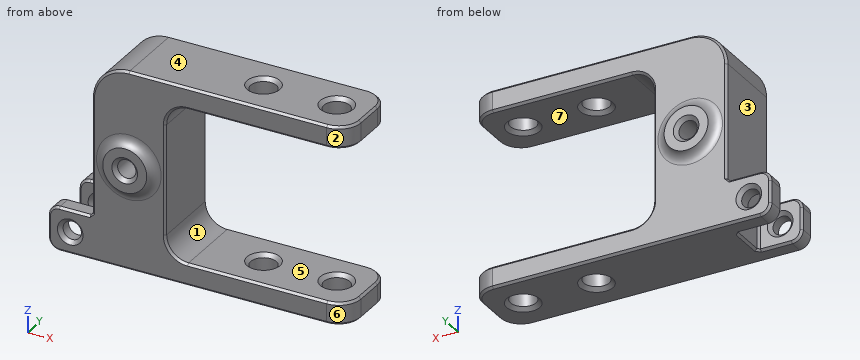
```python
from build123d import *

# Parameters (mm, degrees)
EXTRUDE_1_DEPTH     = 10
SKETCH_2_R          = 1.75
CUT_EXTRUDE_1_DEPTH = 28
SKETCH_3_W          = 6
SKETCH_3_H          = 5.152186346
CUT_EXTRUDE_2_DEPTH = 8
SKETCH_4_R          = 1.25
CUT_EXTRUDE_3_DEPTH = 11
FILLET_1_R          = 3
FILLET_2_R          = 5
FILLET_3_R          = 1.5
SKETCH_5_R          = 3
EXTRUDE_2_DEPTH     = 1
EXTRUDE_START       = 1
SKETCH_6_R          = 3
EXTRUDE_3_DEPTH     = 1
FILLET_4_R          = 1.5
SKETCH_7_R          = 1.25
CUT_EXTRUDE_4_DEPTH = 17
CHAMFER_1_SIZE      = 0.5
FILLET_5_R          = 3
CHAMFER_2_SIZE      = 0.3


with BuildPart() as part:
    # 草图1 → 凸台-拉伸1 (new body)
    with BuildSketch(Plane(origin=(0, 0, 0), x_dir=(1, 0, 0), z_dir=(0, 1, 0))):
        Polygon((23.273216446, 11.883138654), (23.273216446, 8.883138654), (-1.726783554, 8.883138654), (-1.726783554, -12.116861346), (23.273216446, -12.116861346), (23.273216446, -15.116861346), (-11.726783554, -15.116861346), (-11.726783554, 5.883138654), (-17.726783554, 5.883138654), (-17.726783554, 11.883138654), (-11.726783554, 11.883138654), align=None)
    extrude(amount=EXTRUDE_1_DEPTH)

    # 草图2 → 切除-拉伸1 (cut)
    with BuildSketch(Plane(origin=(0, 0, -11.883138654), x_dir=(-1, 0, 0), z_dir=(0, 0, -1))):
        with Locations((-18.858625261, 5)):
            Circle(SKETCH_2_R)
        with Locations((-8.858625261, 5)):
            Circle(SKETCH_2_R)
    extrude(amount=-CUT_EXTRUDE_1_DEPTH, mode=Mode.SUBTRACT)

    # 草图3 → 切除-拉伸2 (cut)
    with BuildSketch(Plane.XY.offset(-5.883138654)):
        with Locations((-14.726783554, 4.923906827)):
            Rectangle(SKETCH_3_W, SKETCH_3_H)
    extrude(amount=-CUT_EXTRUDE_2_DEPTH, mode=Mode.SUBTRACT)

    # 草图4 → 切除-拉伸3 (cut)
    with BuildSketch(Plane(origin=(0, 10, 0), x_dir=(1, 0, 0), z_dir=(0, 1, 0))):
        with Locations(Location((-14.726783554, 8.883138654, 0), (0, 0, 270))):
            Circle(SKETCH_4_R)
    extrude(amount=-CUT_EXTRUDE_3_DEPTH, mode=Mode.SUBTRACT)

    # 圆角1
    fillet_1_edges = [part.edges().sort_by_distance(p)[0] for p in [
        (23.273216446, 0, -10.383138654),
        (23.273216446, 0, 13.616861346),
        (23.273216446, 10, 13.616861346),
        (23.273216446, 10, -10.383138654),
    ]]
    fillet(fillet_1_edges, radius=FILLET_1_R)

    # 圆角2
    fillet_2_edges = [part.edges().sort_by_distance(p)[0] for p in [
        (-11.726783554, 5, 15.116861346),
    ]]
    fillet(fillet_2_edges, radius=FILLET_2_R)

    # 圆角3
    fillet_3_edges = [part.edges().sort_by_distance(p)[0] for p in [
        (-17.726783554, 8.75, -5.883138654),
        (-17.726783554, 8.75, -11.883138654),
        (-17.726783554, 1.173906827, -11.883138654),
        (-17.726783554, 1.173906827, -5.883138654),
    ]]
    fillet(fillet_3_edges, radius=FILLET_3_R)

    # 草图5 → 凸台-拉伸2 (add)
    with BuildSketch(Plane.XZ):
        with Locations(Location((-6.726783554, 2.116861346, 0), (0, 0, 90))):
            Circle(SKETCH_5_R)
    extrude(amount=EXTRUDE_2_DEPTH)

    # 草图6 → 凸台-拉伸3 (add)
    with BuildSketch(Plane(origin=(0, 10, 0), x_dir=(1, 0, 0), z_dir=(0, 1, 0)).offset(EXTRUDE_START)):
        with Locations(Location((-6.726783554, -2.116861346, 0), (0, 0, 270))):
            Circle(SKETCH_6_R)
    extrude(amount=-EXTRUDE_3_DEPTH)

    # 圆角4
    # the kernel refuses this fillet: 1.5 mm, written as the material it adds along each edge
    with BuildSketch(Plane(origin=(-6.726783554, 0, 2.116861346), x_dir=(0, 0, 1), z_dir=(1, 0, 0))) as fillet_4_piece_1:
        with BuildLine():
            CenterArc((4.414213562, 1.5), FILLET_4_R, 199.471220634, 70.528779366)
            Line((3, 1), (2.971715729, 0.99))
            ThreePointArc((2.971715729, 0.99), (2.97, 0.5), (2.97, 0))
            Line((2.97, 0), (3, -0.03))
            Line((3, -0.03), (4.414213562, -0.03))
            Line((4.414213562, -0.03), (4.414213562, 0))
        make_face()
    revolve(axis=Axis((-6.726783554, 0, 2.116861346), (0, -1, 0)))
    with BuildSketch(Plane(origin=(-6.726783554, 10, 2.116861346), x_dir=(0, 0, 1), z_dir=(-1, 0, 0))) as fillet_4_piece_2:
        with BuildLine():
            CenterArc((4.414213562, 1.5), FILLET_4_R, 199.471220634, 70.528779366)
            Line((3, 1), (2.971715729, 0.99))
            ThreePointArc((2.971715729, 0.99), (2.97, 0.5), (2.97, 0))
            Line((2.97, 0), (3, -0.03))
            Line((3, -0.03), (4.414213562, -0.03))
            Line((4.414213562, -0.03), (4.414213562, 0))
        make_face()
    revolve(axis=Axis((-6.726783554, 10, 2.116861346), (0, 1, 0)))

    # 草图7 → 切除-拉伸4 (cut)
    with BuildSketch(Plane.XZ.offset(1)):
        with Locations(Location((-6.726783554, 2.116861346, 0), (0, 0, 270))):
            Circle(SKETCH_7_R)
    extrude(amount=-CUT_EXTRUDE_4_DEPTH, mode=Mode.SUBTRACT)

    # 倒角1
    chamfer_1_edges = [part.edges().sort_by_distance(p)[0] for p in [
        (-6.726783554, 11, 3.366861346),
        (-6.726783554, -1, 3.366861346),
        (20.608625261, 5, 12.116861346),
        (20.608625261, 5, 15.116861346),
        (20.608625261, 5, -8.883138654),
        (20.608625261, 5, -11.883138654),
        (10.608625261, 5, 12.116861346),
        (10.608625261, 5, 15.116861346),
        (10.608625261, 5, -8.883138654),
        (10.608625261, 5, -11.883138654),
        (-14.726783554, 2.347813654, -10.133138654),
        (-14.726783554, 0, -10.133138654),
        (-14.726783554, 7.5, -10.133138654),
        (-14.726783554, 10, -10.133138654),
    ]]
    chamfer(chamfer_1_edges, length=CHAMFER_1_SIZE)

    # 圆角5
    fillet_5_edges = [part.edges().sort_by_distance(p)[0] for p in [
        (-1.726783554, 5, -8.883138654),
        (-1.726783554, 5, 12.116861346),
    ]]
    fillet(fillet_5_edges, radius=FILLET_5_R)

    # 倒角2
    chamfer_2_edges = [part.edges().sort_by_distance(p)[0] for p in [
        (6.773216446, 0, 15.116861346),
        (6.773216446, 10, 15.116861346),
        (-10.26231746, 0, 13.652395252),
        (-10.26231746, 10, 13.652395252),
        (-13.976783554, 10, -5.883138654),
        (-17.726783554, 7.5, -8.883138654),
        (-17.287443726, 7.5, -11.443798826),
        (-17.287443726, 7.5, -6.322478482),
        (-17.726783554, 10, -8.883138654),
        (-17.287443726, 10, -11.443798826),
        (-17.287443726, 10, -6.322478482),
        (-13.976783554, 2.347813654, -5.883138654),
        (-13.976783554, 0, -5.883138654),
        (-17.726783554, 0, -8.883138654),
        (-17.287443726, 0, -11.443798826),
        (-17.287443726, 0, -6.322478482),
        (-17.726783554, 2.347813654, -8.883138654),
        (-13.976783554, 2.347813654, -11.883138654),
        (-17.287443726, 2.347813654, -11.443798826),
        (-17.287443726, 2.347813654, -6.322478482),
        (-11.726783554, 0, 2.116861346),
        (-11.726783554, 10, 2.116861346),
        (-11.726783554, 8.75, -5.883138654),
        (10.773216446, 0, -8.883138654),
        (10.773216446, 10, -8.883138654),
        (-1.726783554, 0, 1.616861346),
        (-1.726783554, 10, 1.616861346),
        (-0.848103898, 0, -8.004458997),
        (-0.848103898, 10, -8.004458997),
        (-0.848103898, 0, 11.23818169),
        (-0.848103898, 10, 11.23818169),
        (-11.726783554, 4.923906827, -11.883138654),
        (-13.976783554, 7.5, -11.883138654),
        (-11.726783554, 1.173906827, -5.883138654),
        (-11.726783554, 7.5, -8.883138654),
        (-11.726783554, 2.347813654, -8.883138654),
        (-13.976783554, 7.5, -5.883138654),
        (23.273216446, 5, 12.116861346),
        (23.273216446, 5, 15.116861346),
        (10.773216446, 0, 12.116861346),
        (10.773216446, 10, 12.116861346),
        (22.394536789, 9.121320344, 12.116861346),
        (22.394536789, 0.878679656, 12.116861346),
        (2.023216446, 0, -11.883138654),
        (22.394536789, 9.121320344, 15.116861346),
        (22.394536789, 0.878679656, 15.116861346),
        (2.023216446, 10, -11.883138654),
        (23.273216446, 5, -11.883138654),
        (23.273216446, 5, -8.883138654),
        (22.394536789, 9.121320344, -11.883138654),
        (22.394536789, 0.878679656, -11.883138654),
        (22.394536789, 9.121320344, -8.883138654),
        (22.394536789, 0.878679656, -8.883138654),
    ]]
    chamfer(chamfer_2_edges, length=CHAMFER_2_SIZE)


solid = part.part
```
The model under review builds one solid part; all positions refer to its coordinate system, in mm. Face numbers are marked on the shaded views. A direction names the side the tool comes from. Round coordinates to 2 decimals unless told otherwise and drop trailing zeros. Order: outer loops, then holes, each group sorted by start corner. A loop starts at its lowest first (then second) coordinate and runs counter-clockwise, first axis right, second up.
(1) Wall thickness on L1, parallel to Z at x = 9, y = 9.5; L2, parallel to X at y = 6, z = 14; L3, parallel to Y at x = 18, z = -9: over which ranges is each line inside the solid? List them lowest first.
Working result:
L1: z = -11.88 to -8.88, 12.12 to 15.12
L2: x = -9.88 to 7.42, 10.29 to 17.42, 20.29 to 23.27
L3: y = 0.18 to 3.05, 6.95 to 9.82
(2) Take a section at A-A, the plane x = 13.5. State the section outline as (y, z) points.
Working result:
outline: (0, -11.58) - (0.3, -11.88) - (9.7, -11.88) - (10, -11.58) - (10, -9.18) - (9.7, -8.88) - (0.3, -8.88) - (0, -9.18) - close; (0, 12.42) - (0.3, 12.12) - (9.7, 12.12) - (10, 12.42) - (10, 14.82) - (9.7, 15.12) - (0.3, 15.12) - (0, 14.82) - close
(3) Mouldability with a two-part tool opening along Z and no side actions: class the marked faces 4, 5, 6 and 7 as released by +Z, released by -Z, zero draft, split by the parting line, or undercut.
Working result:
face 4: released by +Z
face 5: undercut
face 6: zero draft
face 7: undercut
(4) Take a section at B-B, the plane y = 5. Count the separate pieces of the cut face and the enclosed holes in it, plus the area to 3 significant figures.
Working result:
separate pieces: 5
enclosed holes: 1
area: 369 mm2
(5) For P1, Ø1, axis at y = 6.5, z = -8.5, coming from the +X side; P2, Ø2, axis at x = -14.5, y = 8.5, coming from the +Z side; P3, Ø1.6, axis at x = -13.5, z = -9.5, coming from the +Y side, all flat-tipped, find the tip position at first contact; note any pin that passes through.
Working result:
P1: stops at x = 23.09
P2: stops at z = -5.88
P3: stops at y = 10
(6) Tool access review of the marked faces 1, 2 and 3: name each direction out of +Z, -Z, +X, -X, +Y, -Y from which nothing blocks a thin tool from reaching the whole face with its end or side.
Working result:
face 1: +X, +Y, -Y
face 2: +Z, -Z, +X, -Y
face 3: +Z, -X
